from build123d import *

# Parameters (mm, degrees)
F1_DEPTH = 152.4


with BuildPart() as f1:
    # F0 (on Front) → F1 (new body)
    with BuildSketch(Plane.XZ):
        with BuildLine():
            Line((-8.73125, 3.96875), (-8.73125, -3.96875))
            Line((-8.73125, -3.96875), (5.55625, -3.96875))
            Line((5.55625, -3.96875), (5.55625, -2.38125))
            ThreePointArc((5.55625, -2.38125), (7.801314, -1.451314), (8.73125, 0.79375))
            ThreePointArc((8.73125, 0.79375), (7.801314, 3.038814), (5.55625, 3.96875))
            Line((5.55625, 3.96875), (-8.73125, 3.96875))
        make_face()
    extrude(amount=F1_DEPTH)


solid = f1.part
Can you work these out from the model? Positions are in its coordinate system, mm. Round coordinates to 2 decimals unless told otherwise and drop trailing zeros. Loops run counter-clockwise (first coordinate to the right, second up) from the corner with the lowest first, then second, coordinate; pieces in that order, holes last. Notation, with made-up numbers: (45, -28) - (72, -28) arc R16 ccw to (72, -14) - close; hole circle Ø11 at (-7.75, 0.25). An arc over 180 degrees is marked (long way). Use CSV: the item, a comma, the result in double quotes. Start each with the question number.
1) If we section it at B-B on z = -0.75: Write out the boundary of the cut face in (x, y).
2) Please list where these lines run through material, in increasing order: probe 1 along X at (y, z) = (-123, -2.75); probe 2 along Z at (x, y) = (7.25, -95.5); probe 3 along X at (y, z) = (-132.5, -1.25). Write a range as [from, to].
3) If we section it at A-A on y = -30.5: Write out the boundary of the cut face in (x, z) (3 decimals), plus the area to 3 significant figures.
4) If we section it at C-C on x = 7: Write out the boundary of the cut face in (y, z), plus the area to 3 significant figures.
5) For pin 1 Ø0.8 at (y, z) = (-53.5, -3.5) entering from +X; pin 2 Ø3 at (y, z) = (-93.5, -1.5) entering from +X, each with a flat end and sliding along its axis, tell me the tip position at first contact or that it passes through.
Geometry results:
1,outline,"(-8.73, -152.4) - (8.33, -152.4) - (8.33, 0) - (-8.73, 0) - close"
2,probe 1,"x = [-8.73, 5.56]"
2,probe 2,"z = [-1.89, 3.48]"
2,probe 3,"x = [-8.73, 7.99]"
3,outline,"(-8.731, -3.969) - (5.556, -3.969) - (5.556, -2.381) arc R3.175 ccw to (5.556, 3.969) - (-8.731, 3.969) - close"
3,area,"129 mm2"
4,outline,"(-152.4, -2.03) - (0, -2.03) - (0, 3.62) - (-152.4, 3.62) - close"
4,area,"862 mm2"
5,pin 1,"stops at x = 5.56"
5,pin 2,"stops at x = 8.63"
